from build123d import *

# Parameters (mm, degrees)
SKETCH1_R           = 24.455055929
SKETCH1_R_2         = 2.54
BOSS_EXTRUDE1_DEPTH = 5.08
SKETCH4_R           = 30.48
BOSS_EXTRUDE3_DEPTH = 2.54
SKETCH5_R           = 2.54
CUT_EXTRUDE2_DEPTH  = 8.62
SKETCH6_R           = 45.336039437
SKETCH6_R_2         = 37.958395775
BOSS_EXTRUDE4_DEPTH = 2.54
SKETCH7_R           = 2.54
CUT_EXTRUDE3_DEPTH  = 3.54
BOSS_EXTRUDE6_DEPTH = 5.08
SKETCH11_R          = 2.54
CUT_EXTRUDE4_DEPTH  = 8.62


with BuildPart() as part:
    # Sketch1 → Boss-Extrude1 (new body)
    with BuildSketch(Plane.XY):
        with BuildLine():
            Line((-16.891, -131.282672274), (16.891, -131.282672274))
            ThreePointArc((16.891, -131.282672274), (21.504350582, -110.13005032), (34.5064888, -92.819336271))
            ThreePointArc((34.5064888, -92.819336271), (0, 0), (-34.5064888, -92.819336271))
            ThreePointArc((-34.5064888, -92.819336271), (-21.504350582, -110.13005032), (-16.891, -131.282672274))
        make_face()
        with Locations((0, -52.823729134)):
            Circle(SKETCH1_R, mode=Mode.SUBTRACT)
        with Locations((-10.756405179, -114.872047193)):
            Circle(SKETCH1_R_2, mode=Mode.SUBTRACT)
        with Locations((10.756405179, -114.872047193)):
            Circle(SKETCH1_R_2, mode=Mode.SUBTRACT)
    extrude(amount=BOSS_EXTRUDE1_DEPTH)

    # Sketch4 → Boss-Extrude3 (add)
    with BuildSketch(Plane.XY.offset(5.08)):
        with Locations((0, -52.823729134)):
            Circle(SKETCH4_R)
    extrude(amount=BOSS_EXTRUDE3_DEPTH)

    # Sketch5 → Cut-Extrude2 (cut, through all)
    with BuildSketch(Plane.XY.offset(7.62)):
        with Locations((0, -52.823729134)):
            Circle(SKETCH5_R)
    extrude(amount=-CUT_EXTRUDE2_DEPTH, mode=Mode.SUBTRACT)

    # Sketch6 → Boss-Extrude4 (add)
    with BuildSketch(Plane(origin=(0, 0, 0), x_dir=(-1, 0, 0), z_dir=(0, 0, -1))):
        with Locations((0, -52.823729134)):
            Circle(SKETCH6_R)
        with Locations((0, -52.823729134)):
            Circle(SKETCH6_R_2, mode=Mode.SUBTRACT)
        with BuildLine():
            Line((16.891, -131.282672274), (-16.891, -131.282672274))
            ThreePointArc((-16.891, -131.282672274), (-19.272918471, -115.909664076), (-26.19530634, -101.978279981))
            Line((-26.19530634, -101.978279981), (26.19530634, -101.978279981))
            ThreePointArc((26.19530634, -101.978279981), (19.272918471, -115.909664076), (16.891, -131.282672274))
        make_face()
    extrude(amount=BOSS_EXTRUDE4_DEPTH)

    # Sketch7 → Cut-Extrude3 (cut, through all)
    with BuildSketch(Plane.XY):
        with Locations((-10.756405179, -114.872047193)):
            Circle(SKETCH7_R)
        with Locations((10.756405179, -114.872047193)):
            Circle(SKETCH7_R)
    extrude(amount=-CUT_EXTRUDE3_DEPTH, mode=Mode.SUBTRACT)

    # Sketch10 → Boss-Extrude6 (add)
    with BuildSketch(Plane.XY.offset(5.08)):
        with BuildLine():
            add(Edge.make_bspline(
                [(-68.900180003, -24.949874899), (-63.297197231, -26.895437115), (-51.389708048, -24.415182371), (-41.569282444, -19.727412804), (-37.524583334, -15.645079276)],
                knots=[0, 0, 0, 0, 0.520070067, 1, 1, 1, 1], degree=3))
            ThreePointArc((-68.900180003, -24.949874899), (-98.354072, -43.866775297), (-72.9914133, -67.993864183))
            add(Edge.make_bspline(
                [(-72.9914133, -67.993864183), (-65.508215076, -66.903538588), (-55.033388576, -68.640688731), (-47.574313167, -76.247284621), (-45.161811227, -80.223677424)],
                knots=[0, 0, 0, 0, 0.604504859, 1, 1, 1, 1], degree=3))
            ThreePointArc((-45.161811227, -80.223677424), (-52.45816234, -46.619894549), (-37.524583334, -15.645079276))
        make_face()
    extrude(amount=-BOSS_EXTRUDE6_DEPTH)

    # Sketch11 → Cut-Extrude4 (cut, through all)
    with BuildSketch(Plane.XY.offset(5.08)):
        with Locations((-76.2, -45.972469461)):
            Circle(SKETCH11_R)
    extrude(amount=-CUT_EXTRUDE4_DEPTH, mode=Mode.SUBTRACT)


solid = part.part
Read the model definition and answer for the solid it produces. Units are mm, in the model's axes. A direction names the side the tool comes from. Coordinates: 2 decimals unless noted, no trailing zeros. Order: outer loops, then holes, each group sorted by start corner. A loop starts at its lowest first (then second) coordinate and runs counter-clockwise, first axis right, second up. Notation, with made-up numbers: (87, -5) - (128, -5) arc R30 ccw to (128, 31) - close; hole circle Ø3 at (4.25, 15). An arc over 180 degrees is marked (long way). Use one line per item in the form item = value.
(1) Section B-B, the plane y = -85 is taken. Give the vertices of the cut face in (x, z).
Computed values:
outline = (-41.89, 0) - (-31.94, 0) - (-31.94, -2.54) - (-20.14, -2.54) - (-20.14, 0) - (20.14, 0) - (20.14, -2.54) - (31.94, -2.54) - (31.94, 0) - (41.89, 0) - (41.89, 5.08) - (-41.89, 5.08) - close
(2) Given pin 1 Ø8 at (x, y) = (10.76, -114.87) entering from -Z; pin 2 Ø2 at (y, z) = (-48, 0) entering from -X; pin 3 Ø8 at (x, y) = (-76.2, -45.97) entering from +Z; pin 4 Ø3 at (y, z) = (-14, -1) entering from -X, each flat-ended and moving along its own axis, determine where each tip first touches the part or whether it passes through.
Computed values:
pin_1 = -2.54
pin_2 = -98.43
pin_3 = 5.08
pin_4 = -36.99
(3) Which of the six approach directions +Z, -Z, +X, -X, +Y, -Y give full straight-line access (tool end or side, diameter ignored) to faces 4 (the face through (-0.3, -50.3, 6.4)), 5 (the face through (-6.61, -82.58, 6.33)), 6 (the face through (5, -52, 5.08))?
Computed values:
face_4 = +Z, -Z
face_5 = +Z
face_6 = -Z
(4) Section A-A, the plane x = 0 is taken. Give the vertices of the cut face in (y, z), then the cut area to 3 significant figures.
Computed values:
outline = (-131.28, -2.54) - (-101.98, -2.54) - (-101.98, 0) - (-98.16, 0) - (-98.16, -2.54) - (-90.78, -2.54) - (-90.78, 0) - (-77.28, 0) - (-77.28, 5.08) - (-55.36, 5.08) - (-55.36, 7.62) - (-83.3, 7.62) - (-83.3, 5.08) - (-131.28, 5.08) - close; (-50.28, 5.08) - (-28.37, 5.08) - (-28.37, 0) - (-14.87, 0) - (-14.87, -2.54) - (-7.49, -2.54) - (-7.49, 0) - (0, 0) - (0, 5.08) - (-22.34, 5.08) - (-22.34, 7.62) - (-50.28, 7.62) - close
area = 672 mm²
(5) Section C-C, the plane x = -76.2 is taken. Give the vertices of the cut face in (y, z), then the cut area to 3 significant figures.
Computed values:
outline = (-68.23, 0) - (-48.51, 0) - (-48.51, 5.08) - (-68.23, 5.08) - close; (-43.43, 0) - (-23.72, 0) - (-23.72, 5.08) - (-43.43, 5.08) - close
area = 200 mm²
(6) Section D-D, the plane y = -105 is taken. Give the vertices of the cut face in (x, z), then the cut area to 3 significant figures.
Computed values:
outline = (-24.22, -2.54) - (24.22, -2.54) - (24.22, 5.08) - (-24.22, 5.08) - close
area = 369 mm²
(7) For a pull along Y with two mould halves and no side action, classify faces 1 (the face through (-98.294, -43.306, 2.576)), 2 (the face through (4.94, -15.19, -1.25)), 3 (the face through (0, -131.283, 1)) as pulls with the +Y half, pulls with the -Y half, needs draft (parallel to the pull), parting line crosses it, or undercut.
Computed values:
face_1 = parting line crosses it
face_2 = undercut
face_3 = pulls with the -Y half
(8) Straight lines are drawn through the part: L1, parallel to Y at x = 0, z = 1.6; L2, parallel to Y at x = 6.5, z = -1.75; L3, parallel to Y at x = 5.5, z = -1.25. For each, find the intervals that lie inside material, in ascending order.
Computed values:
L1 = -131.28 to -77.28, -28.37 to 0
L2 = -131.28 to -101.98, -97.69 to -90.22, -15.43 to -7.96
L3 = -131.28 to -101.98, -97.82 to -90.38, -15.27 to -7.82
